```python
from build123d import *

# Parameters (mm, degrees)
BOSS_EXTRUDE1_DEPTH      = 250
BOSS_EXTRUDE1_DEPTH_BACK = 200
SKETCH2_W                = 21
SKETCH2_H                = 21
SKETCH3_W                = 16
SKETCH3_H                = 16
CUT_EXTRUDE1_DEPTH       = 800
SKETCH14_R               = 2.5
BOSS_EXTRUDE3_DEPTH      = 10
LPATTERN1_COUNT          = 2
LPATTERN1_PITCH          = 120


with BuildPart() as part:
    # Sketch2 → Boss-Extrude1 (new, two sides: drawn at the far end of the back side and taken through both)
    with BuildSketch(Plane(origin=(0, 0, 0), x_dir=(1, 0, 0), z_dir=(0, 1, 0)).offset(-BOSS_EXTRUDE1_DEPTH_BACK)):
        Rectangle(SKETCH2_W, SKETCH2_H)
    extrude(amount=BOSS_EXTRUDE1_DEPTH + BOSS_EXTRUDE1_DEPTH_BACK)

    # Sketch3 → Cut-Extrude1 (cut)
    with BuildSketch(Plane.XZ.offset(200)):
        Rectangle(SKETCH3_W, SKETCH3_H)
    extrude(amount=-CUT_EXTRUDE1_DEPTH, mode=Mode.SUBTRACT)

    # Sketch14 → Boss-Extrude3 (add)
    with BuildSketch(Plane(origin=(9.15884387, 19.641204062, 19.641204062), x_dir=(0.9497051253149476, -0.22142738646170096, -0.2214273864617029), z_dir=(0.3131456130149675, 0.6715429342378182, 0.6715429342378204))):
        Polygon((-12.902384486, 16.967939861), (98.008310235, -50.846644091), (103.224816692, -42.31505219), (-7.685878028, 25.499531762), align=None)
        with Locations(Location((87.819175611, -38.756088454, 0), (0, 0, 270))):
            Circle(SKETCH14_R, mode=Mode.SUBTRACT)
    boss_extrude3 = extrude(amount=-BOSS_EXTRUDE3_DEPTH)

    # LPattern1: Boss-Extrude3 ×2
    with Locations(*[(0, i * LPATTERN1_PITCH, 0) for i in range(1, LPATTERN1_COUNT)]):
        add(boss_extrude3)


solid = part.part
```
Source: CAD feature listing. Evaluate the final solid. Frame: model axes, mm. A direction names the side the tool comes from. Round coordinates to 2 decimals unless told otherwise and drop trailing zeros. Loops run counter-clockwise (first coordinate to the right, second up) from the corner with the lowest first, then second, coordinate; pieces in that order, holes last.
1. Contact query for flat-ended pins moving along their axis: pin 1 (13 mm diameter, centred on y = -65, z = -2, fed in from +X); pin 2 (10.5 mm diameter, centred on x = 4, y = -22.5, fed in from +Z); pin 3 (5 mm diameter, centred on x = 61.5, z = 13, fed in from +Y). Output: stop coordinate, or through.
2. Mould query, pull axis Z, two halves, no side actions, for faces 5 (the cylindrical face through (88.911, 89.156, 25.596)), 6 (the flat face through (47.29, -4.562, 18.722)), 7 (the flat face through (53.6, -7.89, 11.56)). Classes: released by +Z, released by -Z, zero draft, split by the parting line, or undercut.
3. Ray query, L1, parallel to X at y = 116, z = 2; L2, parallel to Y at x = 16.5, z = 13; L3, parallel to Y at x = 50.5, z = 13.5. Return the intervals inside material, ascending.
4. Section query B-B on y = -3. Output: boundary loops of the cut face in (x, z), and give its area (3 significant figures).
5. Access query for faces 1 (the flat face through (-2.127, 153.659, 3.545)), 2 (the flat face through (-0.015, 145.71, 6.66)), 3 (the flat face through (103.136, 81.079, 27.039)), 4 (the flat face through (0, 22, -8)). Directions: +Z, -Z, +X, -X, +Y, -Y. A direction counts if a zero-diameter tool reaches every point of the face in a straight line with its end or side. Return the directions, or none.
6. Section query C-C on y = 221. Output: boundary loops of the cut face in (x, z), and give its area (3 significant figures).
7. Section query A-A on x = 63. Output: boundary loops of the cut face in (y, z).
Answers below:
1. pin 1: stops at x = 10.5
1. pin 2: stops at z = 10.5
1. pin 3: stops at y = 117.55
2. face 5: undercut
2. face 6: released by +Z
2. face 7: released by -Z
3. L1: x = -10.5 to -8, 8 to 10.5
3. L2: y = 18.28 to 22.86, 138.28 to 142.86
3. L3: y = -8.39 to 4.98, 111.61 to 124.98
4. outline: (-10.5, -10.5) - (10.5, -10.5) - (10.5, 10.5) - (-10.5, 10.5) - close; (38.49, 13.72) - (50.53, 8.1) - (63.41, 16.98) - (51.37, 22.6) - close; hole (-8, -8) - (8, -8) - (8, 8) - (-8, 8) - close
4. area: 364 mm2
5. face 1: +Y
5. face 2: none
5. face 3: +Z, +X
5. face 4: +Y, -Y
6. outline: (-10.5, -10.5) - (10.5, -10.5) - (10.5, 10.5) - (-10.5, 10.5) - close; hole (-8, -8) - (8, -8) - (8, 8) - (-8, 8) - close
6. area: 185 mm2
7. outline: (-19.87, 19.16) - (-11.59, 10.87) - (-2.72, 16.89) - (-11, 25.18) - close; (100.13, 19.16) - (108.41, 10.87) - (117.28, 16.89) - (109, 25.18) - close
